from build123d import *

# Parameters (mm, degrees)
BOSS_EXTRUDE1_DEPTH = 15
SKETCH2_W           = 7
SKETCH2_H           = 7
SKETCH2_R           = 1
BOSS_EXTRUDE2_DEPTH = 3
CUT_EXTRUDE1_DEPTH  = 1.6


with BuildPart() as part:
    # Sketch1 → Boss-Extrude1 (new body)
    with BuildSketch(Plane.XY):
        with BuildLine():
            Line((-10, 0), (-8.5, 0))
            ThreePointArc((-8.5, 0), (0, -8.5), (8.5, 0))
            Line((8.5, 0), (10, 0))
            ThreePointArc((10, 0), (0, -10), (-10, 0))
        make_face()
    extrude(amount=BOSS_EXTRUDE1_DEPTH)

    # Sketch2 → Boss-Extrude2 (add)
    # profile 1 of 2: a face of its own
    with BuildSketch(Plane(origin=(0, 0, 0), x_dir=(1, 0, 0), z_dir=(0, 1, 0))):
        with Locations((-12, -7.5)):
            Rectangle(SKETCH2_W, SKETCH2_H)
        with Locations(Location((-12, -7.5, 0), (0, 0, 270))):
            Circle(SKETCH2_R, mode=Mode.SUBTRACT)
    # profile 2 of 2: a face of its own
    with BuildSketch(Plane(origin=(0, 0, 0), x_dir=(1, 0, 0), z_dir=(0, 1, 0))):
        with Locations((12, -7.514851196)):
            Rectangle(SKETCH2_W, SKETCH2_H)
        with Locations(Location((12, -7.514851196, 0), (0, 0, 270))):
            Circle(SKETCH2_R, mode=Mode.SUBTRACT)
    extrude(amount=-BOSS_EXTRUDE2_DEPTH)

    # Sketch3 → Cut-Extrude1 (cut, symmetric)
    with BuildSketch(Plane(origin=(0, 0, 7.5), x_dir=(-1, 0, 0), z_dir=(0, 0, -1))):
        with BuildLine():
            Line((-9.35, 0), (-8.5, 0))
            ThreePointArc((-8.5, 0), (0, -8.5), (8.5, 0))
            Line((8.5, 0), (9.35, 0))
            ThreePointArc((9.35, 0), (0, -9.35), (-9.35, 0))
        make_face()
    extrude(amount=CUT_EXTRUDE1_DEPTH, both=True, mode=Mode.SUBTRACT)


solid = part.part
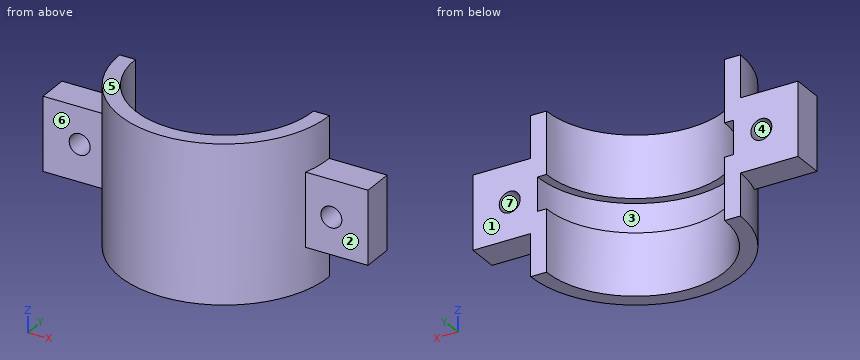
The listing builds one solid part. Answer for the finished solid, in the listing's coordinates (mm). Face numbers are marked on the shaded views. A direction names the side the tool comes from. Coordinates: 2 decimals unless noted, no trailing zeros. Loops run counter-clockwise (first coordinate to the right, second up) from the corner with the lowest first, then second, coordinate; pieces in that order, holes last.
1) A tool of negligible diameter and unlimited length cuts with its end or side. For the marked faces 1, 2 and 3, from which of +Z, -Z, +X, -X, +Y, -Y can it reach the whole face along a straight path? Write none if from no direction.
2) Find section A-A on x = 12. Write down the section's boundary in (y, z).
3) Find the intervals of material crossed by L1, parallel to X at y = -0.95, z = 7.5; L2, parallel to X at y = -6.5, z = 1.5; L3, parallel to X at y = -1.4, z = 7.5, in increasing order.
4) Find section B-B on z = 7.5. Write down the section's boundary in (x, y).
5) Find section D-D on x = 0. Write down the section's boundary in (y, z).
6) Find section C-C on y = -6.5. Write down the section's boundary in (x, z), then the cut area to 3 significant figures.
7) Flat-ended cylindrical pins translate along their axes: pin 1 Ø1.8 at (x, z) = (-12, 7.5) entering from -Y; pin 2 Ø1 at (x, z) = (-2, 11) entering from -Y; pin 3 Ø3 at (x, z) = (-11.5, 11.5) entering from -Y; pin 4 Ø1.5 at (x, y) = (13, -1) entering from -Z. Find the tip coordinate at first contact, or state that the pin passes through.
8) Determine the mould class of the marked faces 4, 5, 6 and 7 for opening direction Z: pulls with the +Z half, pulls with the -Z half, needs draft (parallel to the pull), parting line crosses it, or undercut.
Values:
1. face 1: +Z, -Z, +X, -X, +Y
1. face 2: +Z, -Z, +X, -Y
1. face 3: +Y
2. outline: (-3, 4.01) - (0, 4.01) - (0, 6.51) - (-3, 6.51) - close; (-3, 8.51) - (0, 8.51) - (0, 11.01) - (-3, 11.01) - close
3. L1: x = -15.5 to -13, -11 to -9.3, 9.3 to 11, 13 to 15.5
3. L2: x = -7.6 to -5.48, 5.48 to 7.6
3. L3: x = -15.5 to -13, -11 to -9.24, 9.24 to 11, 13 to 15.5
4. outline: (-15.5, -3) - (-13, -3) - (-13, 0) - (-15.5, 0) - close; (-11, -3) - (-9.54, -3) arc R10 ccw to (9.54, -3) - (11, -3) - (11, 0) - (9.35, 0) arc R9.35 cw to (-9.35, 0) - (-11, 0) - close; (13, -3) - (15.5, -3) - (15.5, 0) - (13, 0) - close
5. outline: (-10, 0) - (-8.5, 0) - (-8.5, 5.9) - (-9.35, 5.9) - (-9.35, 9.1) - (-8.5, 9.1) - (-8.5, 15) - (-10, 15) - close
6. outline: (-7.6, 0) - (-5.48, 0) - (-5.48, 5.9) - (-6.72, 5.9) - (-6.72, 9.1) - (-5.48, 9.1) - (-5.48, 15) - (-7.6, 15) - close; (5.48, 0) - (7.6, 0) - (7.6, 15) - (5.48, 15) - (5.48, 9.1) - (6.72, 9.1) - (6.72, 5.9) - (5.48, 5.9) - close
6. area: 55.7 mm2
7. pin 1: passes through
7. pin 2: stops at y = -9.89
7. pin 3: stops at y = -3
7. pin 4: stops at z = 4.01
8. face 4: undercut
8. face 5: pulls with the +Z half
8. face 6: needs draft
8. face 7: undercut
